For this review, take the finished solid that the model builds, in its own axes (mm). A direction names the side the tool comes from. Round coordinates to 2 decimals unless told otherwise and drop trailing zeros. Order: outer loops, then holes, each group sorted by start corner. A loop starts at its lowest first (then second) coordinate and runs counter-clockwise, first axis right, second up. Notation, with made-up numbers: M -7,58.5 L 52,58.5 A25 cw 52,95.5 Z; hole C -24,-4.5 d3. An arc over 180 degrees is marked long. Answer as a JSON object with one key per item and string values.
from build123d import *

# Parameters (mm, degrees)
F0_W     = 141
F0_H     = 91.5
F0_W_2   = 110
F0_H_2   = 70
F1_DEPTH = 5
F2_DEPTH = 1.25
F3_DEPTH = 5.001
F4_R     = 5
F5_R     = 5


with BuildPart() as f1:
    # F0 (on Front) → F1 (new body, symmetric)
    with BuildSketch(Plane.XZ):
        Polygon((75, 45.5), (75, 55), (-75, 55), (-75, -55), (75, -55), (75, -46), (-66, -46), (-66, 45.5), align=None)
        with Locations((4.5, -0.25)):
            Rectangle(F0_W, F0_H)
        Rectangle(F0_W_2, F0_H_2, mode=Mode.SUBTRACT)
        Rectangle(F0_W_2, F0_H_2)
    extrude(amount=F1_DEPTH, both=True)

    # F0 (on Front) → F2 (cut, symmetric)
    with BuildSketch(Plane.XZ):
        with Locations((4.5, -0.25)):
            Rectangle(F0_W, F0_H)
        Rectangle(F0_W_2, F0_H_2, mode=Mode.SUBTRACT)
        Rectangle(F0_W_2, F0_H_2)
    extrude(amount=F2_DEPTH, both=True, mode=Mode.SUBTRACT)

    # F0 (on Front) → F3 (cut, through all)
    with BuildSketch(Plane.XZ):
        Rectangle(F0_W_2, F0_H_2)
    extrude(amount=F3_DEPTH, mode=Mode.SUBTRACT)

    # F4
    f4_edges = [f1.edges().sort_by_distance(p)[0] for p in [
        (-75, 0, 55),
        (75, 0, 55),
        (75, 0, -55),
        (-75, 0, -55),
    ]]
    fillet(f4_edges, radius=F4_R)

    # F5
    f5_edges = [f1.edges().sort_by_distance(p)[0] for p in [
        (-55, -3.125, 35),
        (55, -3.125, 35),
        (55, -3.125, -35),
        (-55, -3.125, -35),
    ]]
    fillet(f5_edges, radius=F5_R)


solid = f1.part
1) Add section C-C on x = 31.5. State the section outline as (y, z) points, and give its area (3 significant figures).
Geometry check:
{"outline": "M -5,-55 L 5,-55 L 5,55 L -5,55 L -5,35 L -1.25,35 L -1.25,45.5 L 1.25,45.5 L 1.25,-46 L -1.25,-46 L -1.25,-35 L -5,-35 Z", "area": "609 mm²"}
2) Add section A-A on z = 25.5. State the section outline as (x, y) points.
Geometry check:
{"outline": "M -75,-5 L -55,-5 L -55,-1.25 L -66,-1.25 L -66,1.25 L 75,1.25 L 75,5 L -75,5 Z; M 55,-5 L 75,-5 L 75,-1.25 L 55,-1.25 Z"}
3) Add section D-D on z = -38.5. State the section outline as (x, y) points.
Geometry check:
{"outline": "M -75,-5 L 75,-5 L 75,-1.25 L -66,-1.25 L -66,1.25 L 75,1.25 L 75,5 L -75,5 Z"}
4) Machinability: for faces 1 (the flat face through (4, -1.25, -40)), 2 (the cylindrical face through (-54, -3, -33)), 3 (the cylindrical face through (-73, 0, 54)), which of the approach directions +Z, -Z, +X, -X, +Y, -Y give a long, thin tool a straight path to every point of the face, cutting with its end or side? Answer none if there is none.
Geometry check:
{"face 1": "+X", "face 2": "-Y", "face 3": "+Z, -X, +Y, -Y"}
5) Mouldability with a two-part tool opening along X and no side actions: class faces 4 (the cylindrical face through (74, 0, -53)), 5 (the cylindrical face through (53, -3, -34)), 6 (the flat face through (-1, -3, -35)), 7 (the flat face through (-75, 0, 1)) as +X half, -X half, draft (parallel to the pull), parting line (faces both ways), or undercut.
Geometry check:
{"face 4": "+X half", "face 5": "undercut", "face 6": "undercut", "face 7": "-X half"}
6) For L1, parallel to X at y = -1.5, z = -7.5; L2, parallel to Z at x = 6, y = 0.5; L3, parallel to Y at x = 57.5, z = 40, list the stretches that pass through material, from the lowest coordinate up.
Geometry check:
{"L1": "x = -75 to -55, 55 to 75", "L2": "z = -55 to -46, 45.5 to 55", "L3": "y = -5 to -1.25, 1.25 to 5"}
7) Add section B-B on x = 57.5. State the section outline as (y, z) points, and give its area (3 significant figures).
Geometry check:
{"outline": "M -5,-55 L 5,-55 L 5,55 L -5,55 Z; hole M -1.25,-46 L 1.25,-46 L 1.25,45.5 L -1.25,45.5 Z", "area": "871 mm²"}
8) Insertion check: P1, Ø1.2, axis at y = 0.5, z = -20, coming from the +X side; P2, Ø8, axis at x = -24.5, z = 7, coming from the -Y side. Each pin has a flat end and moves straight along its axis. Give the tip position at first contact, or say it passes through.
Geometry check:
{"P1": "stops at x = -66", "P2": "stops at y = 1.25"}
